```python
from build123d import *

# Parameters (mm, degrees)
SKETCH_W     = 8.5
SKETCH_H     = 20.2
PAD_DEPTH    = 15.2
SKETCH001_R  = 1
PAD001_DEPTH = 0.8
SKETCH002_W  = 8.5
SKETCH002_H  = 20.2
PAD002_DEPTH = 3.5
SKETCH003_R  = 4.25
PAD003_DEPTH = 4.5
SKETCH004_R  = 1.85
PAD004_DEPTH = 2.5


with BuildPart() as part:
    # Sketch → Pad (new body)
    with BuildSketch(Plane.XY):
        Rectangle(SKETCH_W, SKETCH_H)
    extrude(amount=PAD_DEPTH)

    # Sketch001 (on Face6 of Pad) → Pad001 (join)
    with BuildSketch(Plane.XY.offset(15.2)):
        Polygon((4.25, 10.1), (4.25, 13.6), (-4.25, 13.6), (-4.25, 10.1), (-4.25, -10.1), (-4.25, -13.6), (4.25, -13.6), (4.25, -10.1), align=None)
        with Locations((0, 11.8)):
            Circle(SKETCH001_R, mode=Mode.SUBTRACT)
        with Locations((0, -11.8)):
            Circle(SKETCH001_R, mode=Mode.SUBTRACT)
    extrude(amount=PAD001_DEPTH)

    # Sketch002 (on Face9 of Pad001) → Pad002 (join)
    with BuildSketch(Plane.XY.offset(16)):
        Rectangle(SKETCH002_W, SKETCH002_H)
    extrude(amount=PAD002_DEPTH)

    # Sketch003 (on Face14 of Pad002) → Pad003 (join)
    with BuildSketch(Plane.XY.offset(19.5)):
        with Locations((0, -5.55)):
            Circle(SKETCH003_R)
    extrude(amount=PAD003_DEPTH)

    # Sketch004 (on Face19 of Pad003) → Pad004 (join)
    with BuildSketch(Plane.XY.offset(24)):
        with Locations((0, -5.55)):
            Circle(SKETCH004_R)
    extrude(amount=PAD004_DEPTH)


solid = part.part
```
The model under review builds one solid part; all positions refer to its coordinate system, in mm. A direction names the side the tool comes from. Give positions to 0.01 mm unless a question says otherwise; leave off trailing zeros. Write each loop counter-clockwise with the first axis right and the second up, starting at its lowest first coordinate (ties: lowest second). Pieces come first, ordered by that corner, then holes. Notation, with made-up numbers: M 40.5,50.25 L 45.5,50.25 A30 ccw 45.5,84.25 Z; hole C -1,11 d5. An arc over 180 degrees is marked long. Write each question's results on one line, items separated by ' | '. Start each with the question number.
1. We need section C-C (x = -3.5). Write out the cut boundary in (y, z).
2. For faces 1 (the flat face through (-1, 11, 16)), 2 (the cylindrical face through (-0.92, -9.7, 21.72)), 3 (the flat face through (-1, -11, 15.2)), 4 (the flat face through (-1, -11, 16)), list the 3-axis set-ups (+Z, -Z, +X, -X, +Y, -Y) from which the entire face can be reached by the end or side of a thin tool; tool diameter is ignored.
3. We need section A-A (x = 0). Write out the cut boundary in (y, z).
4. For probe 1 along Y at (x, z) = (0, 15.8); probe 2 along Y at (x, z) = (2.5, 18); probe 3 along Z at (x, y) = (3, 12), list the stretches that pass through material, from the lowest coordinate up. Write a range as [from, to].
5. We need section B-B (y = -11.8). Write out the cut boundary in (x, z).
6. Mouldability with a two-part tool opening along X and no side actions: class faces 5 (the flat face through (0, -10.1, 7)), 6 (the cylindrical face through (-0.241, -3.716, 25.232)), 7 (the cylindrical face through (-0.13, -10.81, 15.59)) as released by +X, released by -X, zero draft, split by the parting line, or undercut.
7. We need section D-D (y = -6.5). Write out the cut boundary in (x, z), and give its area (3 significant figures).
8. Insertion check: pin 1 Ø1.8 at (x, y) = (0, 11.8) entering from -Z; pin 2 Ø2.5 at (x, z) = (2, 4.5) entering from -Y; pin 3 Ø2.5 at (x, z) = (0.5, 8.5) entering from +Y; pin 4 Ø2.5 at (x, y) = (0, -11.8) entering from +Z. Each pin has a flat end and moves straight along its axis. Give the tip position at first contact, or say it passes through.
Results found:
1) outline: M -13.6,15.2 L -10.1,15.2 L -10.1,0 L 10.1,0 L 10.1,15.2 L 13.6,15.2 L 13.6,16 L 10.1,16 L 10.1,19.5 L -3.14,19.5 L -3.14,24 L -7.96,24 L -7.96,19.5 L -10.1,19.5 L -10.1,16 L -13.6,16 Z
2) face 1: +Z, +X, -X, +Y | face 2: +Z | face 3: -Z, +X, -X, -Y | face 4: +Z, +X, -X, -Y
3) outline: M -13.6,15.2 L -12.8,15.2 L -12.8,16 L -13.6,16 Z; M -10.8,15.2 L -10.1,15.2 L -10.1,0 L 10.1,0 L 10.1,15.2 L 10.8,15.2 L 10.8,16 L 10.1,16 L 10.1,19.5 L -1.3,19.5 L -1.3,24 L -3.7,24 L -3.7,26.5 L -7.4,26.5 L -7.4,24 L -9.8,24 L -9.8,19.5 L -10.1,19.5 L -10.1,16 L -10.8,16 Z; M 12.8,15.2 L 13.6,15.2 L 13.6,16 L 12.8,16 Z
4) probe 1: y = [-13.6, -12.8], [-10.8, 10.8], [12.8, 13.6] | probe 2: y = [-10.1, 10.1] | probe 3: z = [15.2, 16]
5) outline: M -4.25,15.2 L -1,15.2 L -1,16 L -4.25,16 Z; M 1,15.2 L 4.25,15.2 L 4.25,16 L 1,16 Z
6) face 5: zero draft | face 6: split by the parting line | face 7: undercut
7) outline: M -4.25,0 L 4.25,0 L 4.25,19.5 L 4.14,19.5 L 4.14,24 L 1.59,24 L 1.59,26.5 L -1.59,26.5 L -1.59,24 L -4.14,24 L -4.14,19.5 L -4.25,19.5 Z | area: 211 mm^2
8) pin 1: passes through | pin 2: stops at y = -10.1 | pin 3: stops at y = 10.1 | pin 4: stops at z = 16
